```python
from build123d import *

# Parameters (mm, degrees)
BOSS_EXTRUDE1_DEPTH = 6.35
SKETCH2_W           = 19.05
SKETCH2_H           = 190.5
CUT_EXTRUDE1_DEPTH  = 310.869909223
SKETCH3_R           = 4.572
CUT_EXTRUDE2_DEPTH  = 310.869909223


with BuildPart() as part:
    # Sketch1 → Boss-Extrude1 (new body)
    with BuildSketch(Plane(origin=(0, 0, 0), x_dir=(1, 0, 0), z_dir=(0, 1, 0))):
        with BuildLine():
            Line((31.75, -13.073529412), (50.765202328, 17.881902266))
            ThreePointArc((50.765202328, 17.881902266), (55.191250928, 30.365130488), (54.139291827, 43.567943639))
            Line((54.139291827, 43.567943639), (22.722603429, 148.989996692))
            ThreePointArc((22.722603429, 148.989996692), (5.710537817, 226.070917322), (0, 304.8))
            Line((0, 304.8), (-19.05, 304.8))
            Line((-19.05, 304.8), (-19.05, 114.3))
            Line((-19.05, 114.3), (0, 114.3))
            Line((0, 114.3), (0, 0))
            ThreePointArc((0, 0), (11.497376237, -17.168136702), (31.75, -13.073529412))
        make_face()
    extrude(amount=BOSS_EXTRUDE1_DEPTH)

    # Sketch2 → Cut-Extrude1 (cut, through all)
    with BuildSketch(Plane(origin=(0, 6.35, 0), x_dir=(1, 0, 0), z_dir=(0, 1, 0))):
        with Locations((-9.525, 209.55)):
            Rectangle(SKETCH2_W, SKETCH2_H)
    extrude(amount=-CUT_EXTRUDE1_DEPTH, mode=Mode.SUBTRACT)

    # Sketch3 → Cut-Extrude2 (cut, through all)
    with BuildSketch(Plane(origin=(0, 6.35, 0), x_dir=(1, 0, 0), z_dir=(0, 1, 0))):
        with Locations(Location((11.178180871, 46.576310918, 0), (0, 0, 270))):
            Circle(SKETCH3_R)
        with Locations(Location((17.707917982, 9.005992113, 0), (0, 0, 270))):
            Circle(SKETCH3_R)
        with Locations(Location((41.037990009, 18.900486467, 0), (0, 0, 270))):
            Circle(SKETCH3_R)
    extrude(amount=-CUT_EXTRUDE2_DEPTH, mode=Mode.SUBTRACT)


solid = part.part
```
CAD build for the part. Positions are in the model's coordinates, mm. Round coordinates to 2 decimals unless told otherwise and drop trailing zeros. Loops run counter-clockwise (first coordinate to the right, second up) from the corner with the lowest first, then second, coordinate; pieces in that order, holes last. Notation, with made-up numbers: M -35.75,-22 L -27.75,-22 A15 cw -27.75,4 Z; hole C 32,19 d10. An arc over 180 degrees is marked long. Use a Markdown table: item, result. Add a question column.
(1) Drill centre lines: line 1 (X direction, y = 5.5, z = -36.5); line 2 (X direction, y = 3.75, z = -212.5). Where is each one in solid material? Low to high.
(2) Cut at B-B (z = -110.5). Give the cut face in (x, y).
(3) Cut at C-C (z = -216). Give the cut face in (x, y), and give its area (3 significant figures).
(4) Pull direction Z, two halves, no side cores. Call faces 1 (the face through (11.215, 3.131, 17.049)), 2 (the face through (55.166, 3.131, -30.18)), 3 (the face through (9.43, 3.22, -42.35)): +Z half, -Z half, draft (parallel to the pull), parting line (faces both ways), or undercut.
(5) Cut at A-A (y = 4). Give the cut face in (x, z), and give its area (3 significant figures).
(6) Flat gauge pins, fed straight in: pin 1 (7.5 mm diameter, centred on x = 17.71, z = -9.01, fed in from -Y) (3 decimals); pin 2 (2 mm diameter, centred on y = 3, z = -20, fed in from +X). Where does each tip first touch, or does it go through?
Geometry says:
| question | item | result |
|---|---|---|
| 1 | line 1 | x = 0 to 55.4 |
| 1 | line 2 | x = 0 to 7.86 |
| 2 | outline | M 0,0 L 34.19,0 L 34.19,6.35 L 0,6.35 Z |
| 3 | outline | M 0,0 L 7.28,0 L 7.28,6.35 L 0,6.35 Z |
| 3 | area | 46.2 mm² |
| 4 | face 1 | +Z half |
| 4 | face 2 | parting line |
| 4 | face 3 | undercut |
| 5 | outline | M 0,-304.8 A545.56 cw 22.72,-148.99 L 54.14,-43.57 A31.75 ccw 50.77,-17.88 L 31.75,13.07 A18.57 ccw 0,0 Z; hole C 11.18,-46.58 d9.14; hole C 17.71,-9.01 d9.14; hole C 41.04,-18.9 d9.14 |
| 5 | area | 7,780 mm² |
| 6 | pin 1 | passes through |
| 6 | pin 2 | stops at x = 52.45 |
